Here's how the part is built. I have some questions about the finished solid (model axes, mm). Face numbers are marked on the shaded views. A direction names the side the tool comes from. Round coordinates to 2 decimals unless told otherwise and drop trailing zeros. Loops run counter-clockwise (first coordinate to the right, second up) from the corner with the lowest first, then second, coordinate; pieces in that order, holes last. Notation, with made-up numbers: M 22,46.25 L 51,46.25 A10 cw 51,52.25 Z; hole C -14.75,68 d5. An arc over 180 degrees is marked long. Use a Markdown table: item, result.
```python
from build123d import *

# Parameters (mm, degrees)
F1_DEPTH = 63.5
F2_DEPTH = 25.4
F3_DEPTH = 7.9375
F4_DEPTH = 25.4
F6_R     = 6.35


with BuildPart() as f1:
    # F0 (on Front) → F1 (new body, symmetric)
    with BuildSketch(Plane.XZ):
        Polygon((-41.275, 9.525), (-41.275, -9.525), (41.275, -9.525), (41.275, 9.525), (22.225, 9.525), align=None)
    extrude(amount=F1_DEPTH, both=True)

    # F0 (on Front) → F2 (join, symmetric)
    with BuildSketch(Plane.XZ):
        with BuildLine():
            Line((22.225, 9.525), (41.275, 9.525))
            Line((41.275, 9.525), (41.275, 36.848876))
            ThreePointArc((41.275, 36.848876), (47.109768, 49.145598), (60.325, 52.403135))
            Line((60.325, 52.403135), (60.325, 71.4502))
            Line((60.325, 71.4502), (52.406165, 71.4502))
            ThreePointArc((52.406165, 71.4502), (30.830482, 59.806197), (22.225, 36.848876))
            Line((22.225, 36.848876), (22.225, 9.525))
        make_face()
    extrude(amount=F2_DEPTH, both=True)

    # F0 (on Front) → F3 (join, symmetric)
    with BuildSketch(Plane.XZ):
        with BuildLine():
            add(Edge.make_bspline(
                [(-41.275, 9.525), (-39.229893, 47.259647), (12.391411, 67.604472), (52.406165, 71.4502)],
                knots=[0, 0, 0, 0, 112.298224, 112.298224, 112.298224, 112.298224], degree=3))
            Line((-41.275, 9.525), (22.225, 9.525))
            Line((22.225, 9.525), (22.225, 36.848876))
            ThreePointArc((22.225, 36.848876), (30.830482, 59.806197), (52.406165, 71.4502))
        make_face()
    extrude(amount=F3_DEPTH, both=True)

    # F0 (on Front) → F4 (join, symmetric)
    with BuildSketch(Plane.XZ):
        with BuildLine():
            Line((85.725, 71.4502), (60.325, 71.4502))
            Line((60.325, 71.4502), (60.325, 52.403135))
            ThreePointArc((60.325, 52.403135), (60.332174, 52.401669), (60.339347, 52.4002))
            Line((60.339347, 52.4002), (85.725, 52.4002))
            Line((85.725, 52.4002), (85.725, 71.4502))
        make_face()
    extrude(amount=F4_DEPTH, both=True)

    # F0 (on Front) → F5 (revolve)
    with BuildSketch(Plane.XZ):
        Polygon((85.725, 76.2), (85.725, 71.4502), (85.725, 52.4002), (85.725, 47.625), (111.125, 47.625), (111.125, 76.2), align=None)
    revolve(axis=Axis((85.725, 0, 59.5376), (0, 0, -1)))

    # F6
    f6_edges = [f1.edges().sort_by_distance(p)[0] for p in [
        (41.275, -63.5, 0),
        (41.275, 63.5, 0),
        (-41.275, -63.5, 0),
        (-41.275, 63.5, 0),
    ]]
    fillet(f6_edges, radius=F6_R)


solid = f1.part
```
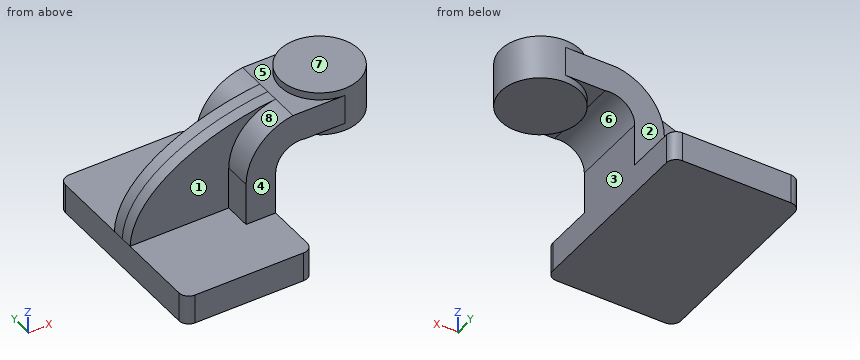
Q1. Imagine slicing it at A-A, the plane z = -1. Please give me the cut outline in (x, y) (3 decimals), then the cut area to 3 significant figures.
Return value:
| item | result |
|---|---|
| outline | M -41.275,-57.15 A6.35 ccw -34.925,-63.5 L 34.925,-63.5 A6.35 ccw 41.275,-57.15 L 41.275,57.15 A6.35 ccw 34.925,63.5 L -34.925,63.5 A6.35 ccw -41.275,57.15 Z |
| area | 10,400 mm^2 |
Q2. I need wall thicknesses on line 1 (Z direction, x = 21, y = 13.5) (3 decimals); line 2 (Y direction, x = 38.5, z = 47.5); line 3 (X direction, y = 13.5, z = 24) (3 decimals). Which ranges of each line are inside material? Lowest first, please. Write a range as from..to.
Return value:
| item | result |
|---|---|
| line 1 | z = -9.525..9.525 |
| line 2 | y = -25.4..25.4 |
| line 3 | x = 22.225..41.275 |
Q3. We'd pull the mould along X, two halves only. Please class the marked faces 6, 7 and 8: pulls with the +X half, pulls with the -X half, needs draft (parallel to the pull), parting line crosses it, or undercut.
Return value:
| item | result |
|---|---|
| face 6 | undercut |
| face 7 | needs draft |
| face 8 | pulls with the -X half |
Q4. For the marked faces 1, 2, 3, 4 and 5, which set-ups out of +Z, -Z, +X, -X, +Y, -Y let a thin tool reach every point of the face, with its end or its side?
Return value:
| item | result |
|---|---|
| face 1 | +Z, -X, -Y |
| face 2 | +Z, +X, -X, +Y |
| face 3 | -Z, +X, +Y, -Y |
| face 4 | +Z, +X, -X, -Y |
| face 5 | +Z, -X |
Q5. Imagine slicing it at C-C, the plane x = 69.5. Please give me the cut outline in (y, z) (1 decimal), then the cut area to 3 significant figures.
Return value:
| item | result |
|---|---|
| outline | M -25.4,52.4 L -19.5,52.4 L -19.5,47.6 L 19.5,47.6 L 19.5,52.4 L 25.4,52.4 L 25.4,71.5 L 19.5,71.5 L 19.5,76.2 L -19.5,76.2 L -19.5,71.5 L -25.4,71.5 Z |
| area | 1,340 mm^2 |
Q6. Imagine slicing it at D-D, the plane y = 40.5. Please give me the cut outline in (x, z) (3 decimals), then the cut area to 3 significant figures.
Return value:
| item | result |
|---|---|
| outline | M -41.275,-9.525 L 41.275,-9.525 L 41.275,9.525 L -41.275,9.525 Z |
| area | 1,570 mm^2 |
Q7. Will these pins go through, and if not, where does the flat tip stop? P1, Ø8.5, axis at y = -21, z = 26.5, coming from the -X side (3 decimals); P2, Ø2, axis at x = 15.5, z = 35, coming from the -Y side; P3, Ø18.5, axis at x = -12.5, z = 34.5, coming from the +Y side; P4, Ø12, axis at y = -34.5, z = 55, coming from the -X side.
Return value:
| item | result |
|---|---|
| P1 | stops at x = 22.225 |
| P2 | stops at y = -7.94 |
| P3 | stops at y = 7.94 |
| P4 | passes through |
Q8. Imagine slicing it at B-B, the plane y = 18.5. Please give me the cut outline in (x, z) (3 decimals).
Return value:
| item | result |
|---|---|
| outline | M -41.275,-9.525 L 41.275,-9.525 L 41.275,36.849 A15.875 cw 60.325,52.403 A17.077 cw 60.339,52.4 L 68.321,52.4 L 68.321,47.625 L 103.129,47.625 L 103.129,76.2 L 68.321,76.2 L 68.321,71.45 L 52.406,71.45 A34.925 ccw 22.225,36.849 L 22.225,9.525 L -41.275,9.525 Z |
